```python
from build123d import *

# Parameters (mm, degrees)
F0_R     = 7.747
F0_R_2   = 11.15
F1_DEPTH = 4.7625
F3_D     = 4.1656


# Not quite as in the source:
# - a feature names something its author has since deleted; it is built from what else it names


with BuildPart() as f1:
    # F0 (on Top) → F1 (new body)
    with BuildSketch(Plane.XY):
        with BuildLine():
            Line((219.054815799, 72.2457910836), (-149.245184201, 72.2457910836))
            ThreePointArc((-149.245184201, 72.2457910836), (-153.7353122615, 70.3859191441), (-155.595184201, 65.8957910836))
            Line((-155.595184201, 65.8957910836), (-155.595184201, -35.7042089164))
            ThreePointArc((-155.595184201, -35.7042089164), (-153.7353122615, -40.194336977), (-149.245184201, -42.0542089164))
            Line((-149.245184201, -42.0542089164), (219.054815799, -42.0542089164))
            ThreePointArc((219.054815799, -42.0542089164), (223.5449438595, -40.194336977), (225.404815799, -35.7042089164))
            Line((225.404815799, -35.7042089164), (225.404815799, 65.8957910836))
            ThreePointArc((225.404815799, 65.8957910836), (223.5449438595, 70.3859191441), (219.054815799, 72.2457910836))
        make_face()
        with BuildLine():
            ThreePointArc((31.9875588712, 4.1757910836), (35.9092220501, 0.923632173), (37.379815799, -3.9542089164))
            ThreePointArc((37.379815799, -3.9542089164), (23.6769747096, -11.3086151675), (25.1220727268, 4.1757910836))
            ThreePointArc((25.1220727268, 4.1757910836), (28.554815799, 4.8707910836), (31.9875588712, 4.1757910836))
        make_face(mode=Mode.SUBTRACT)
        with BuildLine():
            ThreePointArc((82.7875588712, 4.1757910836), (86.7092220501, 0.923632173), (88.179815799, -3.9542089164))
            ThreePointArc((88.179815799, -3.9542089164), (74.4769747096, -11.3086151675), (75.9220727268, 4.1757910836))
            ThreePointArc((75.9220727268, 4.1757910836), (79.354815799, 4.8707910836), (82.7875588712, 4.1757910836))
        make_face(mode=Mode.SUBTRACT)
        with BuildLine():
            ThreePointArc((139.8959807906, 1.2957910836), (141.9937720385, -0.965252677), (142.754815799, -3.9542089164))
            ThreePointArc((142.754815799, -3.9542089164), (133.5158595595, -9.4431651559), (133.1136508074, 1.2957910836))
            ThreePointArc((133.1136508074, 1.2957910836), (136.504815799, 2.2957910836), (139.8959807906, 1.2957910836))
        make_face(mode=Mode.SUBTRACT)
        with BuildLine():
            ThreePointArc((165.2959807906, 1.2957910836), (167.3937720385, -0.965252677), (168.154815799, -3.9542089164))
            ThreePointArc((168.154815799, -3.9542089164), (158.9158595595, -9.4431651559), (158.5136508074, 1.2957910836))
            ThreePointArc((158.5136508074, 1.2957910836), (161.904815799, 2.2957910836), (165.2959807906, 1.2957910836))
        make_face(mode=Mode.SUBTRACT)
        with Locations((-98.445184201, 27.7957910836)):
            Circle(F0_R, mode=Mode.SUBTRACT)
        with Locations((-34.945184201, 27.7957910836)):
            Circle(F0_R, mode=Mode.SUBTRACT)
        with BuildLine():
            ThreePointArc((31.5598116393, 27.5457910836), (34.3286348, 25.0378676617), (35.354815799, 21.4457910836))
            ThreePointArc((35.354815799, 21.4457910836), (24.9627392209, 15.6719720825), (25.5498199587, 27.5457910836))
            ThreePointArc((25.5498199587, 27.5457910836), (28.554815799, 28.2457910836), (31.5598116393, 27.5457910836))
        make_face(mode=Mode.SUBTRACT)
        with BuildLine():
            ThreePointArc((31.5598116393, 52.9457910836), (34.3286348, 50.4378676617), (35.354815799, 46.8457910836))
            ThreePointArc((35.354815799, 46.8457910836), (24.9627392209, 41.0719720825), (25.5498199587, 52.9457910836))
            ThreePointArc((25.5498199587, 52.9457910836), (28.554815799, 53.6457910836), (31.5598116393, 52.9457910836))
        make_face(mode=Mode.SUBTRACT)
        with BuildLine():
            ThreePointArc((82.3533070463, 27.5489910836), (85.1267193187, 25.0409447325), (86.154815799, 21.4457910836))
            ThreePointArc((86.154815799, 21.4457910836), (75.7596621501, 15.6738875639), (76.3563245517, 27.5489910836))
            ThreePointArc((76.3563245517, 27.5489910836), (79.354815799, 28.2457910836), (82.3533070463, 27.5489910836))
        make_face(mode=Mode.SUBTRACT)
        with Locations((193.654815799, 27.7957910836)):
            Circle(F0_R_2, mode=Mode.SUBTRACT)
        with BuildLine():
            ThreePointArc((139.5098116393, 40.2457910836), (142.2786348, 37.7378676617), (143.304815799, 34.1457910836))
            ThreePointArc((143.304815799, 34.1457910836), (132.9127392209, 28.3719720825), (133.4998199587, 40.2457910836))
            ThreePointArc((133.4998199587, 40.2457910836), (136.504815799, 40.9457910836), (139.5098116393, 40.2457910836))
        make_face(mode=Mode.SUBTRACT)
        with BuildLine():
            ThreePointArc((82.3533070463, 52.9489910836), (85.1267193187, 50.4409447325), (86.154815799, 46.8457910836))
            ThreePointArc((86.154815799, 46.8457910836), (75.7596621501, 41.0738875639), (76.3563245517, 52.9489910836))
            ThreePointArc((76.3563245517, 52.9489910836), (79.354815799, 53.6457910836), (82.3533070463, 52.9489910836))
        make_face(mode=Mode.SUBTRACT)
        with BuildLine():
            Line((158.5136508074, 1.2957910836), (165.2959807906, 1.2957910836))
            ThreePointArc((165.2959807906, 1.2957910836), (161.904815799, 2.2957910836), (158.5136508074, 1.2957910836))
        make_face()
        with BuildLine():
            Line((133.1136508074, 1.2957910836), (139.8959807906, 1.2957910836))
            ThreePointArc((139.8959807906, 1.2957910836), (136.504815799, 2.2957910836), (133.1136508074, 1.2957910836))
        make_face()
        with BuildLine():
            Line((25.1220727268, 4.1757910836), (31.9875588712, 4.1757910836))
            ThreePointArc((31.9875588712, 4.1757910836), (28.554815799, 4.8707910836), (25.1220727268, 4.1757910836))
        make_face()
        with BuildLine():
            Line((75.9220727268, 4.1757910836), (82.7875588712, 4.1757910836))
            ThreePointArc((82.7875588712, 4.1757910836), (79.354815799, 4.8707910836), (75.9220727268, 4.1757910836))
        make_face()
        with BuildLine():
            Line((133.4998199587, 40.2457910836), (139.5098116393, 40.2457910836))
            ThreePointArc((139.5098116393, 40.2457910836), (136.504815799, 40.9457910836), (133.4998199587, 40.2457910836))
        make_face()
        with BuildLine():
            Line((25.5498199587, 52.9457910836), (31.5598116393, 52.9457910836))
            ThreePointArc((31.5598116393, 52.9457910836), (28.554815799, 53.6457910836), (25.5498199587, 52.9457910836))
        make_face()
        with BuildLine():
            Line((76.3563245517, 52.9489910836), (82.3533070463, 52.9489910836))
            ThreePointArc((82.3533070463, 52.9489910836), (79.354815799, 53.6457910836), (76.3563245517, 52.9489910836))
        make_face()
        with BuildLine():
            Line((76.3563245517, 27.5489910836), (82.3533070463, 27.5489910836))
            ThreePointArc((82.3533070463, 27.5489910836), (79.354815799, 28.2457910836), (76.3563245517, 27.5489910836))
        make_face()
        with BuildLine():
            Line((25.5498199587, 27.5457910836), (31.5598116393, 27.5457910836))
            ThreePointArc((31.5598116393, 27.5457910836), (28.554815799, 28.2457910836), (25.5498199587, 27.5457910836))
        make_face()
    extrude(amount=F1_DEPTH)

    # F3 (through all)
    with Locations(Plane.XY.offset(4.7625)):
        with Locations((-149.245184201, 65.8957910836), (-149.245184201, -35.7042089164), (219.054815799, 65.8957910836), (219.054815799, -35.7042089164), (-96.667184201, 65.8957910836), (113.644815799, 65.8957910836), (61.066815799, 65.8957910836), (166.222815799, 65.8957910836), (8.488815799, 65.8957910836), (-44.089184201, 65.8957910836), (-149.245184201, -1.6682089164), (-149.245184201, 32.1137910836), (61.066815799, -35.7042089164), (166.222815799, -35.7042089164), (-96.667184201, -35.7042089164), (-44.089184201, -35.7042089164), (113.644815799, -35.7042089164), (8.488815799, -35.7042089164), (219.054815799, -1.9222089164), (219.054815799, 32.1137910836)):
            Hole(F3_D / 2)


solid = f1.part
```
Geometry: final body of the model. Coordinates: model frame, mm. Coordinates: 2 decimals unless noted, no trailing zeros. Write item = value, one per line.
(1) Pin query (flat end, axial travel): pin 1 Ø5.5 at (x, y) = (-44.09, -35.7) entering from +Z. Return the tip coordinate at first contact, or that it passes through.
Solved:
pin_1 = 4.76
(2) Line query: line 1 (Y direction, x = -35.5, z = 0.45); line 2 (X direction, y = -5, z = 0.9); line 3 (X direction, y = 39, z = 1). Output: solid intervals per line, ascending.
Solved:
line_1 = -42.05 to 20.07, 35.52 to 72.25
line_2 = -155.6 to 19.79, 37.32 to 70.59, 88.12 to 130.34, 142.67 to 155.74, 168.07 to 225.4
line_3 = -155.6 to 131.74, 141.27 to 225.4
(3) Cut plane A-A on z = 2.25. Count the separate pieces of the cut face and the enclosed holes in it, plus the area to 3 significant figures.
Solved:
separate_pieces = 1
enclosed_holes = 32
area = 41,000 mm²
(4) Pull-direction query (X, two-part tool) for faces 1 (the cylindrical face through (-40.655, 33.032, 2.348)), 2 (the cylindrical face through (223.5, -40.24, 2.35)), 3 (the cylindrical face through (-153.686, 70.435, 2.348)); classes: pulls with the +X half, pulls with the -X half, needs draft (parallel to the pull), parting line crosses it, or undercut.
Solved:
face_1 = undercut
face_2 = pulls with the +X half
face_3 = pulls with the -X half
